Design review of the part built by this model. Coordinates are the model's own, in mm. Face numbers are marked on the shaded views. A direction names the side the tool comes from. Give positions to 0.01 mm unless a question says otherwise; leave off trailing zeros. Write each question's results on one line, items separated by ' | '. Start each with the question number.
(1) Mouldability with a two-part tool opening along X and no side actions: class the marked faces 1, 2 and 3 as released by +X, released by -X, zero draft, split by the parting line, or undercut.
(2) Take a section at A-A (z = -22). Count the separate pieces of the cut face and the enclosed holes in it, plus the area to 3 significant figures.
(3) For the marked faces 4 and 5, list the 3-axis set-ups (+Z, -Z, +X, -X, +Y, -Y) from which the entire face can be reached by the end or side of a thin tool; tool diameter is ignored.
(4) To check wall thickness, follow probe 1 along X at (y, z) = (12, -11); probe 2 along X at (y, z) = (23, -27.5); probe 3 along Y at (x, z) = (144, -42). State the ranges of each line that lie inside material, in increasing order.
(5) Clearance check with flat-ended pins moving along their axes: pin 1 (4.5 mm diameter, centred on y = 73, z = -37, fed in from -X); pin 2 (1 mm diameter, centred on x = 187, y = 78, fed in from +Z); pin 3 (1.2 mm diameter, centred on x = 114.5, y = 36, fed in from -Z); pin 4 (3 mm diameter, centred on y = 16, z = -36.5, fed in from +X). State where each tip first meets the part, or that it passes through.
from build123d import *

# Parameters (mm, degrees)
BOSS_EXTRUDE1_DEPTH = 120
EXTRUDE_THIN1_DEPTH = 3
LPATTERN2_COUNT     = 16
LPATTERN2_PITCH     = 7


with BuildPart() as part:
    # Sketch1 → Boss-Extrude1 (new body)
    with BuildSketch(Plane(origin=(0, 0, 0), x_dir=(1, 0, 0), z_dir=(0, 1, 0))):
        with BuildLine():
            Line((0, 0), (13, 0))
            ThreePointArc((13, 0), (38, 25), (63, 0))
            Line((63, 0), (78, 0))
            ThreePointArc((78, 0), (103, 25), (128, 0))
            Line((128, 0), (143, 0))
            ThreePointArc((143, 0), (168, 25), (193, 0))
            Line((193, 0), (208, 0))
            ThreePointArc((208, 0), (233, 25), (258, 0))
            Line((258, 0), (271, 0))
            Line((271, 0), (271, 55))
            ThreePointArc((271, 55), (268.071067812, 62.071067812), (261, 65))
            Line((261, 65), (10, 65))
            ThreePointArc((10, 65), (2.928932188, 62.071067812), (0, 55))
            Line((0, 55), (0, 0))
        make_face()
    extrude(amount=BOSS_EXTRUDE1_DEPTH)

    # Sketch3 → Extrude-Thin1 (add)
    with BuildSketch(Plane.XZ):
        with BuildLine():
            Line((274, 0), (274, -55))
            ThreePointArc((274, -55), (270.192388155, -64.192388155), (261, -68))
            Line((261, -68), (10, -68))
            ThreePointArc((10, -68), (0.807611845, -64.192388155), (-3, -55))
            Line((-3, -55), (-3, 0))
            Line((-3, 0), (7, 0))
            Line((7, 0), (7, -55))
            ThreePointArc((7, -55), (7.878679656, -57.121320344), (10, -58))
            Line((10, -58), (261, -58))
            ThreePointArc((261, -58), (263.121320344, -57.121320344), (264, -55))
            Line((264, -55), (264, 0))
            Line((264, 0), (274, 0))
        make_face()
    extrude_thin1 = extrude(amount=EXTRUDE_THIN1_DEPTH)

    # LPattern2: Extrude-Thin1 ×16
    with Locations(*[(0, i * LPATTERN2_PITCH, 0) for i in range(1, LPATTERN2_COUNT)]):
        add(extrude_thin1)


solid = part.part
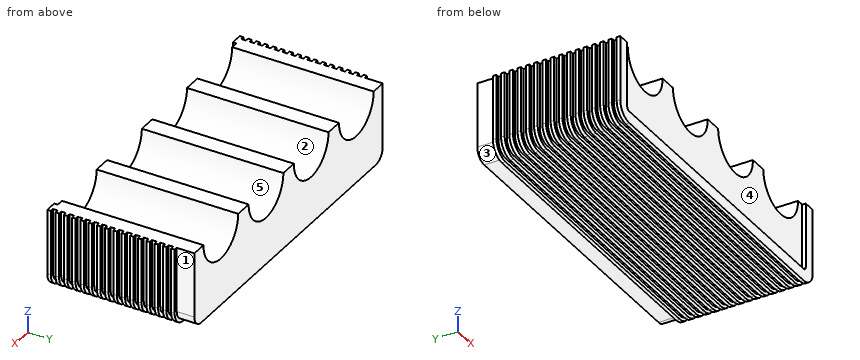
Report:
1) face 1: released by +X | face 2: undercut | face 3: released by -X
2) separate pieces: 5 | enclosed holes: 0 | area: 21,500 mm2
3) face 4: +Z, -Y | face 5: +Z, +Y, -Y
4) probe 1: -3 to 15.55, 60.45 to 80.55, 125.45 to 145.55, 190.45 to 210.55, 255.45 to 274 | probe 2: 0 to 271 | probe 3: 0 to 120
5) pin 1: x = -3 | pin 2: z = -15.64 | pin 3: z = -65 | pin 4: x = 271
